Could you check a few things on this model? Use its own coordinates, in mm. A direction names the side the tool comes from. Give positions to 0.01 mm unless a question says otherwise; leave off trailing zeros. Loops run counter-clockwise (first coordinate to the right, second up) from the corner with the lowest first, then second, coordinate; pieces in that order, holes last. Notation, with made-up numbers: M 38,-14 L 91,-14 A9 ccw 91,-10 Z; hole C 53,-15.75 d5. An arc over 180 degrees is marked long. Use CSV: the item, a comma, the result in double quotes.
```python
from build123d import *

# Parameters (mm, degrees)
BOSS_EXTRUDE1_DEPTH                            = 69.85
CBORE_FOR_4_SOCKET_HEAD_CAP_SCREW1_D           = 3.2639
CBORE_FOR_4_SOCKET_HEAD_CAP_SCREW1_DEPTH       = 9.525
CBORE_FOR_4_SOCKET_HEAD_CAP_SCREW1_CBORE_D     = 3.96875
CBORE_FOR_4_SOCKET_HEAD_CAP_SCREW1_CBORE_DEPTH = 4.7625
CBORE_FOR_4_SOCKET_HEAD_CAP_SCREW1_TIP         = 0.980574487
SKETCH4_R                                      = 2.032
CUT_EXTRUDE1_DEPTH                             = 4.7625
SKETCH5_R                                      = 1.63195
CUT_EXTRUDE2_DEPTH                             = 3.175
CUT_EXTRUDE3_REACH                             = 168.013
SKETCH6_W                                      = 44.45
SKETCH6_H                                      = 31.75


with BuildPart() as part:
    # Sketch1 → Boss-Extrude1 (new body)
    with BuildSketch(Plane(origin=(0, 0, 0), x_dir=(1, 0, 0), z_dir=(0, 1, 0))):
        Polygon((0, 0), (85.725, 0), (85.725, -9.525), (9.525, -9.525), (9.525, -123.825), (0, -123.825), align=None)
    extrude(amount=BOSS_EXTRUDE1_DEPTH)

    # CBORE for #4 Socket Head Cap Screw1
    with Locations(Plane(origin=(0, 0, 0), x_dir=(-1, 0, 0), z_dir=(0, -1, 0))):
        with Locations((-4.7625, -4.7625), (-4.7625, -39.6875), (-4.7625, -74.6125), (-39.6875, -4.7625), (-74.6125, -4.7625), (-4.7625, -109.5375)):
            CounterBoreHole(CBORE_FOR_4_SOCKET_HEAD_CAP_SCREW1_D / 2, CBORE_FOR_4_SOCKET_HEAD_CAP_SCREW1_CBORE_D / 2, CBORE_FOR_4_SOCKET_HEAD_CAP_SCREW1_CBORE_DEPTH, depth=CBORE_FOR_4_SOCKET_HEAD_CAP_SCREW1_DEPTH)
            with Locations((0, 0, -(CBORE_FOR_4_SOCKET_HEAD_CAP_SCREW1_DEPTH + CBORE_FOR_4_SOCKET_HEAD_CAP_SCREW1_TIP / 2))):  # 118° drill point
                Cone(0, CBORE_FOR_4_SOCKET_HEAD_CAP_SCREW1_D / 2, CBORE_FOR_4_SOCKET_HEAD_CAP_SCREW1_TIP, mode=Mode.SUBTRACT)

    # Sketch4 → Cut-Extrude1 (cut)
    with BuildSketch(Plane(origin=(0, 69.85, 0), x_dir=(1, 0, 0), z_dir=(0, 1, 0))):
        with Locations(Location((4.7625, -4.7625, 0), (0, 0, 270))):
            Circle(SKETCH4_R)
        with Locations(Location((80.9625, -4.7625, 0), (0, 0, 270))):
            Circle(SKETCH4_R)
        with Locations(Location((4.7625, -71.4375, 0), (0, 0, 270))):
            Circle(SKETCH4_R)
    extrude(amount=-CUT_EXTRUDE1_DEPTH, mode=Mode.SUBTRACT)

    # Sketch5 → Cut-Extrude2 (cut)
    with BuildSketch(Plane(origin=(0, 65.0875, 0), x_dir=(1, 0, 0), z_dir=(0, 1, 0))):
        with Locations(Location((4.7625, -4.7625, 0), (0, 0, 90))):
            Circle(SKETCH5_R)
        with Locations(Location((80.9625, -4.7625, 0), (0, 0, 270))):
            Circle(SKETCH5_R)
        with Locations(Location((4.7625, -71.4375, 0), (0, 0, 270))):
            Circle(SKETCH5_R)
    extrude(amount=-CUT_EXTRUDE2_DEPTH, mode=Mode.SUBTRACT)

    # Sketch6 → Cut-Extrude3 (cut, up to next)
    with BuildSketch(Plane.ZY, mode=Mode.PRIVATE) as cut_extrude3_sk1:
        with Locations((101.6, 53.975)):
            Rectangle(SKETCH6_W, SKETCH6_H)
    cut_extrude3_tool1 = extrude(cut_extrude3_sk1.sketch, amount=-CUT_EXTRUDE3_REACH, mode=Mode.PRIVATE) & part.part
    add(cut_extrude3_tool1.solids().sort_by_distance((0, 53.975, 101.6))[0], mode=Mode.SUBTRACT)


solid = part.part
```
1. I want a section at A-A, the plane y = 7.5. List the corners of the cut face in (x, z) for me (1 decimal).
Outcome:
outline,"M 0,0 L 85.7,0 L 85.7,9.5 L 9.5,9.5 L 9.5,123.8 L 0,123.8 Z; hole C 4.8,4.8 d3.3; hole C 4.8,39.7 d3.3; hole C 4.8,74.6 d3.3; hole C 4.8,109.5 d3.3; hole C 39.7,4.8 d3.3; hole C 74.6,4.8 d3.3"
2. I'm going to push flat-ended pins straight in: pin 1 Ø3 at (x, z) = (3, 108) entering from +Y; pin 2 Ø2 at (x, z) = (5, 71) entering from +Y; pin 3 Ø2 at (x, y) = (69.5, 54.5) entering from +Z (3 decimals). Where does each tip first touch, or does it pass through?
Outcome:
pin 1,"y = 38.1"
pin 2,"y = 61.91"
pin 3,"z = 9.525"
3. Which directions (+Z, -Z, +X, -X, +Y, -Y) give clear straight access to the entire face, cutting with the end or side of a thin tool? Please do faces 4 (the face through (4.55, 7.177, 72.994)), 5 (the face through (82.58, 63.52, 4.55)), 6 (the face through (0, 34, 49)), 7 (the face through (5, 54, 79.375)).
Outcome:
face 4,"-Y"
face 5,"+Y"
face 6,"+Z, -Z, -X, +Y, -Y"
face 7,"+Z, +X, -X, +Y"
4. I want a section at B-B, the plane x = 57. List the corners of the cut face in (y, z) for me (3 decimals).
Outcome:
outline,"M 0,0 L 69.85,0 L 69.85,9.525 L 0,9.525 Z"
5. I want a section at C-C, the plane y = 42. List the corners of the cut face in (x, z) for me (3 decimals), then the cut area to 3 significant figures.
Outcome:
outline,"M 0,0 L 85.725,0 L 85.725,9.525 L 9.525,9.525 L 9.525,79.375 L 0,79.375 Z"
area,"1,480 mm2"
6. I want a section at D-D, the plane z = 55.5. List the corners of the cut face in (x, y) for me (3 decimals), then the cut area to 3 significant figures.
Outcome:
outline,"M 0,0 L 9.525,0 L 9.525,69.85 L 0,69.85 Z"
area,"665 mm2"
7. If we mould it in two halves opening along X, with no side actions, what happens to faces 1 (the face through (85.725, 34, 5)), 2 (the face through (5, 38.1, 101)), 3 (the face through (81, 61.913, 5))? For each: +X half, -X half, draft (parallel to the pull), parting line (faces both ways), or undercut.
Outcome:
face 1,"+X half"
face 2,"draft"
face 3,"undercut"
8. Please list where this line runs through material, in increasing order: line 1 (X direction, y = 42, z = 49.5) (3 decimals).
Outcome:
line 1,"0 to 9.525"
